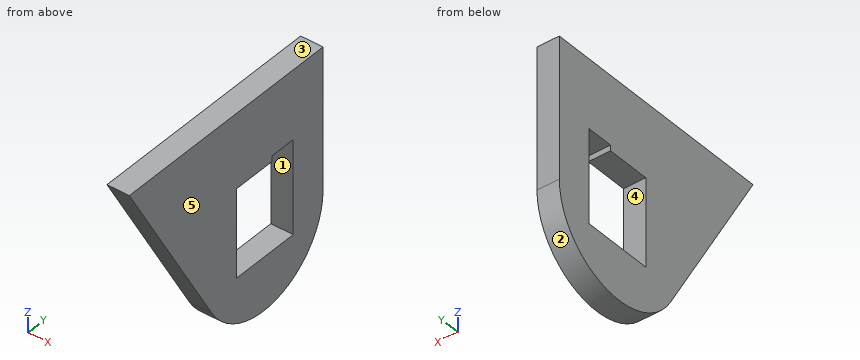
```python
from build123d import *

# Parameters (mm, degrees)
F1_DEPTH = 6


with BuildPart() as f1:
    # F0 (on Right) → F1 (new body)
    with BuildSketch(Plane.YZ):
        with BuildLine():
            Line((87.968563, -69.082131), (22.968563, -69.082131))
            Line((22.968563, -69.082131), (50.648055, -117.024417))
            ThreePointArc((50.648055, -117.024417), (73.144944, -126.342933), (87.968563, -107.024417))
            Line((87.968563, -107.024417), (87.968563, -69.082131))
        make_face()
        Polygon((58.968563, -112.782131), (58.968563, -89.082131), (70.768563, -89.082131), (70.768563, -87.582131), (77.968563, -87.582131), (77.968563, -112.782131), align=None, mode=Mode.SUBTRACT)
    extrude(amount=F1_DEPTH)


solid = f1.part
```
Source: CAD feature listing. Evaluate the final solid. Frame: model axes, mm. Face numbers are marked on the shaded views. A direction names the side the tool comes from. Round coordinates to 2 decimals unless told otherwise and drop trailing zeros. Loops run counter-clockwise (first coordinate to the right, second up) from the corner with the lowest first, then second, coordinate; pieces in that order, holes last. Notation, with made-up numbers: M -3.5,-35 L 8.5,-35 A23 cw 8.5,-8 Z; hole C 79,73.5 d9. An arc over 180 degrees is marked long. Use a Markdown table: item, result. Add a question column.
1. Ray query, line 1 along Y through (x, z) = (0.4, -91); line 2 along Z through (x, y) = (5.3, 61); line 3 along Y through (x, z) = (4.35, -110.5). Return the intervals inside material, ascending. Write a range as [from, to].
2. Pull-direction query (Z, two-part tool) for the marked faces 1, 2 and 3; classes: +Z half, -Z half, draft (parallel to the pull), parting line (faces both ways), or undercut.
3. Cut plane B-B, the plane y = 63.5. Output: boundary loops of the cut face in (x, z).
4. Cut plane A-A, the plane x = 2.8. Output: boundary loops of the cut face in (y, z), and give its area (3 significant figures).
5. Set-up query: the marked faces 4 and 5. Return all of +Z, -Z, +X, -X, +Y, -Y with unobstructed straight access to the full face (end or side cutting, diameter ignored); none if empty.
6. Cut plane D-D, the plane z = -80. Output: boundary loops of the cut face in (x, y).
7. Contact query for flat-ended pins moving along their axis: pin 1 (3 mm diameter, centred on x = 3, z = -104, fed in from -Y); pin 2 (1.8 mm diameter, centred on x = 3, y = 63.5, fed in from -Z); pin 3 (1.5 mm diameter, centred on x = 3.5, z = -110, fed in from +Y). Output: stop coordinate, or through.
8. Cut plane C-C, the plane z = -108.5. Output: boundary loops of the cut face in (x, y), and give its area (3 significant figures).
Solution:
| question | item | result |
|---|---|---|
| 1 | line 1 | y = [35.62, 58.97], [77.97, 87.97] |
| 1 | line 2 | z = [-125.77, -112.78], [-89.08, -69.08] |
| 1 | line 3 | y = [46.88, 58.97], [77.97, 87.66] |
| 2 | face 1 | undercut |
| 2 | face 2 | -Z half |
| 2 | face 3 | +Z half |
| 3 | outline | M 0,-126.52 L 6,-126.52 L 6,-112.78 L 0,-112.78 Z; M 0,-89.08 L 6,-89.08 L 6,-69.08 L 0,-69.08 Z |
| 4 | outline | M 22.97,-69.08 L 50.65,-117.02 A20 ccw 87.97,-107.02 L 87.97,-69.08 Z; hole M 58.97,-112.78 L 77.97,-112.78 L 77.97,-87.58 L 70.77,-87.58 L 70.77,-89.08 L 58.97,-89.08 Z |
| 4 | area | 2,230 mm2 |
| 5 | face 4 | +X, -X |
| 5 | face 5 | +Z, -Z, +X, +Y, -Y |
| 6 | outline | M 0,29.27 L 6,29.27 L 6,87.97 L 0,87.97 Z |
| 7 | pin 1 | stops at y = 42.26 |
| 7 | pin 2 | stops at z = -126.7 |
| 7 | pin 3 | stops at y = 87.84 |
| 8 | outline | M 0,45.73 L 6,45.73 L 6,58.97 L 0,58.97 Z; M 0,77.97 L 6,77.97 L 6,87.91 L 0,87.91 Z |
| 8 | area | 139 mm2 |
